Could you check a few things on this model? Use its own coordinates, in mm. A direction names the side the tool comes from. Give positions to 0.01 mm unless a question says otherwise; leave off trailing zeros. Order: outer loops, then holes, each group sorted by start corner. A loop starts at its lowest first (then second) coordinate and runs counter-clockwise, first axis right, second up.
from build123d import *

# Parameters (mm, degrees)
BOSS_EXTRUDE1_DEPTH = 38
FILLET1_R           = 4
FILLET2_R           = 4
FILLET3_RADIUS      = 19
FILLET3_LENGTH      = 1.7
CUT_EXTRUDE1_DEPTH  = 38
SKETCH3_R           = 2
CUT_EXTRUDE2_DEPTH  = 38
FILLET4_R           = 2


with BuildPart() as part:
    # Sketch1 → Boss-Extrude1 (new body)
    with BuildSketch(Plane.XY):
        Polygon((0, 0), (0, 39), (1.7, 39), (1.7, -1.7), (-49.3, -1.7), (-49.3, 0), align=None)
    extrude(amount=BOSS_EXTRUDE1_DEPTH)

    # Fillet1
    fillet1_edges = [part.edges().sort_by_distance(p)[0] for p in [
        (-49.3, -0.85, 0),
    ]]
    fillet(fillet1_edges, radius=FILLET1_R)

    # Fillet2
    fillet2_edges = [part.edges().sort_by_distance(p)[0] for p in [
        (-49.3, -0.85, 38),
    ]]
    fillet(fillet2_edges, radius=FILLET2_R)

    # Fillet3: full round fillet: the end face becomes a half cylinder, R = half its width
    fillet3_face = Plane((0.85, 39, 19), x_dir=(1, 0, 0), z_dir=(0, 1, 0))  # on the end face: x along it, z out of the body
    fillet3_slab = fillet3_face.offset(-FILLET3_RADIUS / 2) * Box(FILLET3_LENGTH, 2 * FILLET3_RADIUS, FILLET3_RADIUS, mode=Mode.PRIVATE)  # the body's end, R deep
    fillet3_round = Plane((0.85, 20, 19), x_dir=(0, 1, 0), z_dir=(1, 0, 0)) * Cylinder(FILLET3_RADIUS, FILLET3_LENGTH, mode=Mode.PRIVATE)  # its axis R under the face
    add(fillet3_slab - fillet3_round, mode=Mode.SUBTRACT)

    # Sketch2 → Cut-Extrude1 (cut)
    with BuildSketch(Plane(origin=(1.7, 0, 0), x_dir=(0, 0, -1), z_dir=(1, 0, 0))):
        with BuildLine():
            Line((-25.5, 12.013917936), (-25.5, 27.1))
            ThreePointArc((-25.5, 27.1), (-19, 33.6), (-12.5, 27.1))
            Line((-12.5, 27.1), (-12.5, 12.013917936))
            ThreePointArc((-12.5, 12.013917936), (-19, 5.513917936), (-25.5, 12.013917936))
        make_face()
    extrude(amount=-CUT_EXTRUDE1_DEPTH, mode=Mode.SUBTRACT)

    # Sketch3 → Cut-Extrude2 (cut)
    with BuildSketch(Plane(origin=(0, -1.7, 0), x_dir=(-1, 0, 0), z_dir=(0, -1, 0))):
        with Locations(Location((44.7, -3, 0), (0, 0, 180))):
            Circle(SKETCH3_R)
        with Locations(Location((25.7, -3, 0), (0, 0, 180))):
            Circle(SKETCH3_R)
        with Locations(Location((6.7, -3, 0), (0, 0, 180))):
            Circle(SKETCH3_R)
        with Locations(Location((6.7, -35, 0), (0, 0, 90))):
            Circle(SKETCH3_R)
        with Locations(Location((25.7, -35, 0), (0, 0, 90))):
            Circle(SKETCH3_R)
        with Locations(Location((44.7, -35, 0), (0, 0, 90))):
            Circle(SKETCH3_R)
    extrude(amount=-CUT_EXTRUDE2_DEPTH, mode=Mode.SUBTRACT)

    # Fillet4
    fillet4_edges = [part.edges().sort_by_distance(p)[0] for p in [
        (1.7, -1.7, 19),
    ]]
    fillet(fillet4_edges, radius=FILLET4_R)


solid = part.part
Item 1: Imagine slicing it at C-C on y = 7. List the corners of the cut face in (x, z) for me.
Findings:
outline: (0, 0) - (1.7, 0) - (1.7, 14.86) - (0, 14.86) - close; (0, 23.14) - (1.7, 23.14) - (1.7, 38) - (0, 38) - close
Item 2: Imagine slicing it at A-A on x = -6.7. List the corners of the cut face in (y, z) for me.
Findings:
outline: (-1.7, 0) - (0, 0) - (0, 1) - (-1.7, 1) - close; (-1.7, 5) - (0, 5) - (0, 33) - (-1.7, 33) - close; (-1.7, 37) - (0, 37) - (0, 38) - (-1.7, 38) - close
Item 3: We'd pull the mould along Y, two halves only. Please class faces 4 (the flat face through (-14.7, -0.4, 38)), 5 (the cylindrical face through (1.1, -1.13, 19.27)), 6 (the flat face through (1, 19, 25.5)): +Y half, -Y half, draft (parallel to the pull), parting line (faces both ways), or undercut.
Findings:
face 4: draft
face 5: -Y half
face 6: undercut
Item 4: For faces 1 (the flat face through (-25, 0, 19)), 2 (the flat face through (1, 20, 12.5)), 3 (the cylindrical face through (-48.159, -0.838, 1.203)), which set-ups out of +Z, -Z, +X, -X, +Y, -Y let a thin tool reach every point of the face, with its end or its side?
Findings:
face 1: +Z, -Z, -X, +Y
face 2: +X, -X
face 3: -Z, -X, +Y, -Y
Item 5: For pin 1 (8 mm diameter, centred on x = -17.5, z = 16.5, fed in from +Y); pin 2 (1 mm diameter, centred on y = 23, z = 11, fed in from -X); pin 3 (1.4 mm diameter, centred on x = 1, y = 22.5, fed in from +Z), each with a flat end and sliding along its axis, tell me the tip position at first contact or that it passes through.
Findings:
pin 1: stops at y = 0
pin 2: stops at x = 0
pin 3: stops at z = 37.91
Item 6: Imagine slicing it at D-D on z = 3. List the corners of the cut face in (x, y) for me, then the cut area to 3 significant figures.
Findings:
outline: (-49.17, -1.7) - (-46.7, -1.7) - (-46.7, 0) - (-49.17, 0) - close; (-42.7, -1.7) - (-27.7, -1.7) - (-27.7, 0) - (-42.7, 0) - close; (-23.7, -1.7) - (-8.7, -1.7) - (-8.7, 0) - (-23.7, 0) - close; (-4.7, -1.7) - (-0.3, -1.7) arc R2 ccw to (1.7, 0.3) - (1.7, 30.25) - (0, 30.25) - (0, 0) - (-4.7, 0) - close
area: 117 mm2
Item 7: Please list where these lines run through material, in increasing order: line 1 along X through (y, z) = (-0.7, 35); line 2 along Z through (x, y) = (-6, -1); line 3 along Y through (x, z) = (-47, 14.5).
Findings:
line 1: x = -49.17 to -46.7, -42.7 to -27.7, -23.7 to -8.7, -4.7 to 1.43
line 2: z = 0 to 1.13, 4.87 to 33.13, 36.87 to 38
line 3: y = -1.7 to 0
Item 8: Imagine slicing it at B-B on z = 19. List the corners of the cut face in (x, y) for me.
Findings:
outline: (-49.3, -1.7) - (-0.3, -1.7) arc R2 ccw to (1.7, 0.3) - (1.7, 5.51) - (0, 5.51) - (0, 0) - (-49.3, 0) - close; (0, 33.6) - (1.7, 33.6) - (1.7, 39) - (0, 39) - close
